from build123d import *

# Parameters (mm, degrees)
SKETCH1_W               = 44
SKETCH1_H               = 277
SKETCH1_W_2             = 6
SKETCH1_H_2             = 9
SKETCH1_W_3             = 9.5
SKETCH1_H_3             = 6
BOSS_EXTRUDE1_DEPTH     = 6
CUT_EXTRUDE1_DEPTH      = 288.445647036
CUT_EXTRUDE1_DEPTH_BACK = 288.445647036
SKETCH2_R               = 4.5
SKETCH2_R_2             = 2.75
SKETCH2_W               = 11
SKETCH2_H               = 20
CUT_EXTRUDE3_DEPTH      = 288.445647036
CUT_EXTRUDE3_DEPTH_BACK = 288.445647036
SKETCH4_R               = 2.5
CUT_EXTRUDE4_DEPTH      = 288.445647036
CUT_EXTRUDE4_DEPTH_BACK = 288.445647036
SKETCH5_R               = 1.6


with BuildPart() as part:
    # Sketch1 → Boss-Extrude1 (new body)
    with BuildSketch(Plane(origin=(0, 0, 0), x_dir=(1, 0, 0), z_dir=(0, 1, 0))):
        with Locations((22, 138.5)):
            Rectangle(SKETCH1_W, SKETCH1_H)
        with Locations((-3, 12)):
            Rectangle(SKETCH1_W_2, SKETCH1_H_2)
        with Locations((-3, 32)):
            Rectangle(SKETCH1_W_2, SKETCH1_H_2)
        with Locations((-3, 52)):
            Rectangle(SKETCH1_W_2, SKETCH1_H_2)
        with Locations((-3, 72)):
            Rectangle(SKETCH1_W_2, SKETCH1_H_2)
        with Locations((-3, 92)):
            Rectangle(SKETCH1_W_2, SKETCH1_H_2)
        with Locations((-3, 112)):
            Rectangle(SKETCH1_W_2, SKETCH1_H_2)
        with Locations((-3, 132)):
            Rectangle(SKETCH1_W_2, SKETCH1_H_2)
        with Locations((-3, 152)):
            Rectangle(SKETCH1_W_2, SKETCH1_H_2)
        with Locations((-3, 172)):
            Rectangle(SKETCH1_W_2, SKETCH1_H_2)
        with Locations((-3, 192)):
            Rectangle(SKETCH1_W_2, SKETCH1_H_2)
        with Locations((-3, 212)):
            Rectangle(SKETCH1_W_2, SKETCH1_H_2)
        with Locations((-3, 232)):
            Rectangle(SKETCH1_W_2, SKETCH1_H_2)
        with Locations((-3, 252)):
            Rectangle(SKETCH1_W_2, SKETCH1_H_2)
        with Locations((-3, 272)):
            Rectangle(SKETCH1_W_2, SKETCH1_H_2)
        with Locations((12, 280)):
            Rectangle(SKETCH1_W_3, SKETCH1_H_3)
        with Locations((32, 280)):
            Rectangle(SKETCH1_W_3, SKETCH1_H_3)
        with Locations((47, 272)):
            Rectangle(SKETCH1_W_2, SKETCH1_H_2)
        with Locations((47, 252)):
            Rectangle(SKETCH1_W_2, SKETCH1_H_2)
        with Locations((47, 232)):
            Rectangle(SKETCH1_W_2, SKETCH1_H_2)
        with Locations((47, 212)):
            Rectangle(SKETCH1_W_2, SKETCH1_H_2)
        with Locations((47, 192)):
            Rectangle(SKETCH1_W_2, SKETCH1_H_2)
        with Locations((47, 172)):
            Rectangle(SKETCH1_W_2, SKETCH1_H_2)
        with Locations((47, 152)):
            Rectangle(SKETCH1_W_2, SKETCH1_H_2)
        with Locations((47, 132)):
            Rectangle(SKETCH1_W_2, SKETCH1_H_2)
        with Locations((47, 112)):
            Rectangle(SKETCH1_W_2, SKETCH1_H_2)
        with Locations((47, 92)):
            Rectangle(SKETCH1_W_2, SKETCH1_H_2)
        with Locations((47, 72)):
            Rectangle(SKETCH1_W_2, SKETCH1_H_2)
        with Locations((47, 52)):
            Rectangle(SKETCH1_W_2, SKETCH1_H_2)
        with Locations((47, 32)):
            Rectangle(SKETCH1_W_2, SKETCH1_H_2)
        with Locations((47, 12)):
            Rectangle(SKETCH1_W_2, SKETCH1_H_2)
    extrude(amount=BOSS_EXTRUDE1_DEPTH)

    # Sketch2 → Cut-Extrude1 (cut, two sides: drawn at the far end of the back side and taken through both)
    with BuildSketch(Plane(origin=(0, 6, 0), x_dir=(1, 0, 0), z_dir=(0, 1, 0)).offset(-CUT_EXTRUDE1_DEPTH_BACK)):
        with Locations(Location((22, 267, 0), (0, 0, 270))):
            Circle(SKETCH2_R)
        with Locations(Location((22, 227, 0), (0, 0, 270))):
            Circle(SKETCH2_R)
        with Locations(Location((6, 227, 0), (0, 0, 270))):
            Circle(SKETCH2_R_2)
        with Locations(Location((38, 227, 0), (0, 0, 270))):
            Circle(SKETCH2_R_2)
        with Locations((22, 247)):
            Rectangle(SKETCH2_W, SKETCH2_H)
    extrude(amount=CUT_EXTRUDE1_DEPTH + CUT_EXTRUDE1_DEPTH_BACK, mode=Mode.SUBTRACT)

    # Sketch4 → Cut-Extrude3 (cut, two sides: drawn at the far end of the back side and taken through both)
    with BuildSketch(Plane(origin=(0, 6, 0), x_dir=(1, 0, 0), z_dir=(0, 1, 0)).offset(-CUT_EXTRUDE3_DEPTH_BACK)):
        with Locations(Location((33, 39, 0), (0, 0, 270))):
            Circle(SKETCH4_R)
        with Locations(Location((11, 39, 0), (0, 0, 270))):
            Circle(SKETCH4_R)
    extrude(amount=CUT_EXTRUDE3_DEPTH + CUT_EXTRUDE3_DEPTH_BACK, mode=Mode.SUBTRACT)

    # Sketch5 → Cut-Extrude4 (cut, two sides: drawn at the far end of the back side and taken through both)
    with BuildSketch(Plane(origin=(0, 6, 0), x_dir=(1, 0, 0), z_dir=(0, 1, 0)).offset(-CUT_EXTRUDE4_DEPTH_BACK)):
        with Locations(Location((-3, 12, 0), (0, 0, 270))):
            Circle(SKETCH5_R)
        with Locations(Location((47, 12, 0), (0, 0, 270))):
            Circle(SKETCH5_R)
        with Locations(Location((47, 52, 0), (0, 0, 270))):
            Circle(SKETCH5_R)
        with Locations(Location((47, 92, 0), (0, 0, 270))):
            Circle(SKETCH5_R)
        with Locations(Location((47, 132, 0), (0, 0, 270))):
            Circle(SKETCH5_R)
        with Locations(Location((47, 172, 0), (0, 0, 270))):
            Circle(SKETCH5_R)
        with Locations(Location((47, 212, 0), (0, 0, 270))):
            Circle(SKETCH5_R)
        with Locations(Location((-3, 52, 0), (0, 0, 270))):
            Circle(SKETCH5_R)
        with Locations(Location((-3, 92, 0), (0, 0, 270))):
            Circle(SKETCH5_R)
        with Locations(Location((-3, 132, 0), (0, 0, 270))):
            Circle(SKETCH5_R)
        with Locations(Location((-3, 172, 0), (0, 0, 270))):
            Circle(SKETCH5_R)
        with Locations(Location((-3, 212, 0), (0, 0, 270))):
            Circle(SKETCH5_R)
        with Locations(Location((32, 280, 0), (0, 0, 270))):
            Circle(SKETCH5_R)
        with Locations(Location((12, 280, 0), (0, 0, 270))):
            Circle(SKETCH5_R)
    extrude(amount=CUT_EXTRUDE4_DEPTH + CUT_EXTRUDE4_DEPTH_BACK, mode=Mode.SUBTRACT)


solid = part.part
Source: CAD feature listing. Evaluate the final solid. Frame: model axes, mm. A direction names the side the tool comes from. Coordinates: 2 decimals unless noted, no trailing zeros. Loops run counter-clockwise (first coordinate to the right, second up) from the corner with the lowest first, then second, coordinate; pieces in that order, holes last. Notation, with made-up numbers: (8.5, 67) - (46.5, 67) arc R33 cw to (46.5, 97) - close; hole circle Ø2 at (60.25, 46.5). An arc over 180 degrees is marked (long way). One line per item, written item: value. Start each with the question number.
1. Section A-A (z = -242.5). Return the cut outline in (x, y).
2. Mould query, pull axis X, two halves, no side actions, for faces 1 (the flat face through (0, 3, -62)), 2 (the flat face through (50, 3, -132)), 3 (the cylindrical face through (38.83, 2.96, -224.38)). Classes: pulls with the +X half, pulls with the -X half, needs draft (parallel to the pull), parting line crosses it, or undercut.
3. Section B-B (y = 1.5). State how many separate pieces and enclosed holes the cut face has, and give its area (3 significant figures).
4. Contact query for flat-ended pins moving along their axis: P1, Ø1.8, axis at x = 48, y = 4, coming from the +Z side; P2, Ø1.8, axis at y = 4, z = -81.5, coming from the -X side; P3, Ø1.5, axis at y = 4.5, z = -40, coming from the +X side. Output: stop coordinate, or through.
5. Set-up query: faces 4 (the flat face through (-3, 3, -27.5)), 5 (the flat face through (47, 3, -87.5)), 6 (the flat face through (47, 3, -276.5)), 7 (the flat face through (27.25, 3, -280)), 8 (the flat face through (16.5, 3, -247)). Return all of +Z, -Z, +X, -X, +Y, -Y with unobstructed straight access to the full face (end or side cutting, diameter ignored); none if empty.
6. Section C-C (z = -205). Return the cut outline in (x, y).
7. Ray query, L1, parallel to X at y = 2.15, z = -52; L2, parallel to X at y = 3.3, z = -39; L3, parallel to Z at x = 32, y = 3.2. Return the intervals inside material, ascending.
Verdict:
1. outline: (0, 0) - (16.5, 0) - (16.5, 6) - (0, 6) - close; (27.5, 0) - (44, 0) - (44, 6) - (27.5, 6) - close
2. face 1: pulls with the -X half
2. face 2: pulls with the +X half
2. face 3: undercut
3. separate pieces: 1
3. enclosed holes: 21
3. area: 13,300 mm2
4. P1: stops at z = -7.5
4. P2: stops at x = 0
4. P3: stops at x = 44
5. face 4: -X, +Y, -Y
5. face 5: +X, +Y, -Y
5. face 6: -Z, +X, +Y, -Y
5. face 7: -Z, +Y, -Y
5. face 8: +Y, -Y
6. outline: (0, 0) - (44, 0) - (44, 6) - (0, 6) - close
7. L1: x = -6 to -4.6, -1.4 to 45.4, 48.6 to 50
7. L2: x = 0 to 8.5, 13.5 to 30.5, 35.5 to 44
7. L3: z = -283 to -281.6, -278.4 to -41.29, -36.71 to 0
